from build123d import *

# Parameters (mm, degrees)
F0_R     = 8
F0_R_2   = 7.875
F0_R_3   = 0.675
F0_R_4   = 3
F0_R_5   = 2
F0_R_6   = 1
F1_DEPTH = 25.4
F2_DEPTH = 6.5
F3_DEPTH = 0.7
F4_DEPTH = 1.35
F5_DEPTH = 4
F6_R     = 1
F7_DEPTH = 5
F6_R_2   = 2.5
F8_DEPTH = 1.85


# Not quite as in the source:
# - after a boolean that leaves OpenCascade's solid faulty, fix() repairs it


with BuildPart() as f1:
    # F0 (on Right) → F1 (new body)
    with BuildSketch(Plane.YZ):
        Circle(F0_R)
        Circle(F0_R_2, mode=Mode.SUBTRACT)
        Circle(F0_R_2)
        with Locations((-4.3301270189, -2.5)):
            Circle(F0_R_3, mode=Mode.SUBTRACT)
        with Locations((4.3301270189, -2.5)):
            Circle(F0_R_3, mode=Mode.SUBTRACT)
        Circle(F0_R_4, mode=Mode.SUBTRACT)
        with Locations((0, 5)):
            Circle(F0_R_3, mode=Mode.SUBTRACT)
        Circle(F0_R_4)
        Circle(F0_R_5, mode=Mode.SUBTRACT)
        Circle(F0_R_5)
        Circle(F0_R_6, mode=Mode.SUBTRACT)
        Circle(F0_R_6)
        with Locations((0, 5)):
            Circle(F0_R_3)
        with Locations((4.3301270189, -2.5)):
            Circle(F0_R_3)
        with Locations((-4.3301270189, -2.5)):
            Circle(F0_R_3)
    extrude(amount=-F1_DEPTH)

    # F0 (on Right) → F2 (join)
    with BuildSketch(Plane.YZ):
        Circle(F0_R_6)
    extrude(amount=F2_DEPTH)

    # F0 (on Right) → F3 (join)
    with BuildSketch(Plane.YZ):
        Circle(F0_R_4)
        Circle(F0_R_5, mode=Mode.SUBTRACT)
    extrude(amount=F3_DEPTH)

    # F0 (on Right) → F4 (cut)
    with BuildSketch(Plane.YZ):
        with Locations((0, 5)):
            Circle(F0_R_3)
        with Locations((4.3301270189, -2.5)):
            Circle(F0_R_3)
        with Locations((-4.3301270189, -2.5)):
            Circle(F0_R_3)
    extrude(amount=-F4_DEPTH, mode=Mode.SUBTRACT)

    # F0 (on Right) → F5 (cut)
    with BuildSketch(Plane.YZ):
        Circle(F0_R)
        Circle(F0_R_2, mode=Mode.SUBTRACT)
    extrude(amount=-F5_DEPTH, mode=Mode.SUBTRACT)

    # F6 (on face) → F7 (join)
    with BuildSketch(Plane(origin=(-25.4, 0, 0), x_dir=(0, -1, 0), z_dir=(-1, 0, 0))):
        Circle(F6_R)
    extrude(amount=F7_DEPTH)

    # F6 (on face) → F8 (join)
    with BuildSketch(Plane(origin=(-25.4, 0, 0), x_dir=(0, -1, 0), z_dir=(-1, 0, 0))):
        Circle(F6_R_2)
        Circle(F6_R, mode=Mode.SUBTRACT)
        with BuildLine():
            ThreePointArc((8, 0), (7.8992004853, 1.2659509046), (7.5993420768, 2.5))
            Line((7.5993420768, 2.5), (5.75, 2.5))
            Line((5.75, 2.5), (5.75, -2.5))
            Line((5.75, -2.5), (7.5993420768, -2.5))
            ThreePointArc((7.5993420768, -2.5), (7.8992004853, -1.2659509046), (8, 0))
        make_face()
        with BuildLine():
            Line((-5.75, 2.5), (-7.5993420768, 2.5))
            ThreePointArc((-7.5993420768, 2.5), (-8, 0), (-7.5993420768, -2.5))
            Line((-7.5993420768, -2.5), (-5.75, -2.5))
            Line((-5.75, -2.5), (-5.75, 2.5))
        make_face()
    extrude(amount=F8_DEPTH)

    add(f1.part.fix(), mode=Mode.REPLACE)


solid = f1.part
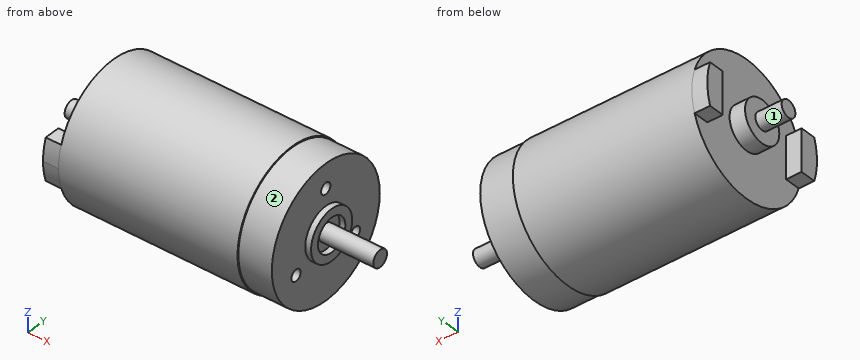
Verification items for the finished model (mm, model axes). Face numbers are marked on the shaded views. A direction names the side the tool comes from. Coordinates: 2 decimals unless noted, no trailing zeros. Loops run counter-clockwise (first coordinate to the right, second up) from the corner with the lowest first, then second, coordinate; pieces in that order, holes last. Notation, with made-up numbers: (-3.75, 52) -> (10.25, 52) arc R24 ccw to (10.25, 89) -> close; hole circle Ø6 at (25.25, 66). An arc over 180 degrees is marked (long way). Answer as a JSON object with one key per item and string values. Group by question number.
Item 1: Sectioned sample at D-D on y = -6.25. Record the boundary of the cut face in (x, z).
Item 2: Tool access check on the marked faces 1 and 2. Record the directions out of +Z, -Z, +X, -X, +Y, -Y that give a thin tool (end or side, any length) a straight path to the whole face; none if there is none.
Item 3: Scan lines: probe 1 along X at (y, z) = (2.5, -4.25); probe 2 along X at (y, z) = (7.5, -2); probe 3 along Y at (x, z) = (-24, -0.25). Record each from-to range of solid material in increasing order.
Item 4: Sectioned sample at C-C on z = -5. Record the boundary of the cut face in (x, y) (3 decimals).
Item 5: Depth check by flat-ended pin: pin 1 (1.1 mm diameter, centred on y = -4.5, z = -2.5, fed in from +X); pin 2 (4 mm diameter, centred on x = -26.5, y = 2.5, fed in from +Z); pin 3 (0.9 mm diameter, centred on x = -26.5, y = 6.5, fed in from -Z). Enter the tip coordinate at first touch or a pass-through.
Item 6: Sectioned sample at B-B on x = -3. Record the boundary of the cut face in (y, z) (3 decimals).
Evaluation:
{
 "1": {"outline": "(-27.25, -2.5) -> (-25.4, -2.5) -> (-25.4, -4.99) -> (-4, -4.99) -> (-4, -4.79) -> (0, -4.79) -> (0, 4.79) -> (-4, 4.79) -> (-4, 4.99) -> (-25.4, 4.99) -> (-25.4, 2.5) -> (-27.25, 2.5) -> close"},
 "2": {"face 1": "-X", "face 2": "+X"},
 "3": {"probe 1": "x = -25.4 to 0", "probe 2": "x = -27.25 to 0", "probe 3": "y = -8 to 8"},
 "4": {"outline": "(-25.4, -6.245) -> (-4, -6.245) -> (-4, -6.084) -> (0, -6.084) -> (0, 6.084) -> (-4, 6.084) -> (-4, 6.245) -> (-25.4, 6.245) -> close"},
 "5": {"pin 1": "stops at x = 0", "pin 2": "stops at z = 7.96", "pin 3": "stops at z = -2.5"},
 "6": {"outline": "circle Ø15.75 at (0, 0)"}
}
